```python
from build123d import *

# Parameters (mm, degrees)
F0_R     = 14
F1_DEPTH = 32
F2_DEPTH = 10
F3_D     = 16
F3_DEPTH = 50
F3_TIP   = 4.8068849522
F4_D     = 16
F4_DEPTH = 50
F4_TIP   = 4.8068849522


with BuildPart() as f1:
    # F0 (on Front) → F1 (new body)
    with BuildSketch(Plane.XZ):
        Circle(F0_R)
    extrude(amount=-F1_DEPTH)

    # F0 (on Front) → F2 (join)
    with BuildSketch(Plane.XZ):
        with BuildLine():
            Line((20, -13.2664991614), (20, 13.2664991614))
            ThreePointArc((20, 13.2664991614), (0, 24), (-20, 13.2664991614))
            Line((-20, 13.2664991614), (-20, -13.2664991614))
            ThreePointArc((-20, -13.2664991614), (0, -24), (20, -13.2664991614))
        make_face()
        with BuildLine():
            ThreePointArc((15.2337502822, 11.3548602959), (18.0338744501, 5.981586104), (19, 0))
            ThreePointArc((19, 0), (18.0338744501, -5.981586104), (15.2337502822, -11.3548602959))
            ThreePointArc((15.2337502822, -11.3548602959), (15.9359270771, -12.2913470597), (16.1850288425, -13.4350288425))
            ThreePointArc((16.1850288425, -13.4350288425), (14.3947257991, -16.0121360874), (11.3548602959, -15.2337502822))
            ThreePointArc((11.3548602959, -15.2337502822), (7.2709852149, -17.5537111177), (2.7427894128, -18.8009868421))
            ThreePointArc((2.7427894128, -18.8009868421), (2.748196762, -18.9004281295), (2.75, -19))
            ThreePointArc((2.75, -19), (-0.0995718705, -21.748196762), (-2.7427894128, -18.8009868421))
            ThreePointArc((-2.7427894128, -18.8009868421), (-7.2709852149, -17.5537111177), (-11.3548602959, -15.2337502822))
            ThreePointArc((-11.3548602959, -15.2337502822), (-15.3795724908, -15.3795724908), (-15.2337502822, -11.3548602959))
            ThreePointArc((-15.2337502822, -11.3548602959), (-19, 0), (-15.2337502822, 11.3548602959))
            ThreePointArc((-15.2337502822, 11.3548602959), (-15.3795724908, 15.3795724908), (-11.3548602959, 15.2337502822))
            ThreePointArc((-11.3548602959, 15.2337502822), (-7.2709852149, 17.5537111177), (-2.7427894128, 18.8009868421))
            ThreePointArc((-2.7427894128, 18.8009868421), (-0.0995718705, 21.748196762), (2.75, 19))
            ThreePointArc((2.75, 19), (2.748196762, 18.9004281295), (2.7427894128, 18.8009868421))
            ThreePointArc((2.7427894128, 18.8009868421), (7.2709852149, 17.5537111177), (11.3548602959, 15.2337502822))
            ThreePointArc((11.3548602959, 15.2337502822), (14.3947257991, 16.0121360874), (16.1850288425, 13.4350288425))
            ThreePointArc((16.1850288425, 13.4350288425), (15.9359270771, 12.2913470597), (15.2337502822, 11.3548602959))
        make_face(mode=Mode.SUBTRACT)
        with BuildLine():
            ThreePointArc((15.2337502822, -11.3548602959), (18.0338744501, -5.981586104), (19, 0))
            ThreePointArc((19, 0), (18.0338744501, 5.981586104), (15.2337502822, 11.3548602959))
            ThreePointArc((15.2337502822, 11.3548602959), (11.4904851943, 11.4904851943), (11.3548602959, 15.2337502822))
            ThreePointArc((11.3548602959, 15.2337502822), (7.2709852149, 17.5537111177), (2.7427894128, 18.8009868421))
            ThreePointArc((2.7427894128, 18.8009868421), (0, 16.25), (-2.7427894128, 18.8009868421))
            ThreePointArc((-2.7427894128, 18.8009868421), (-7.2709852149, 17.5537111177), (-11.3548602959, 15.2337502822))
            ThreePointArc((-11.3548602959, 15.2337502822), (-10.8579215977, 14.3947257991), (-10.6850288425, 13.4350288425))
            ThreePointArc((-10.6850288425, 13.4350288425), (-12.2913470597, 10.934130608), (-15.2337502822, 11.3548602959))
            ThreePointArc((-15.2337502822, 11.3548602959), (-19, 0), (-15.2337502822, -11.3548602959))
            ThreePointArc((-15.2337502822, -11.3548602959), (-12.2913470597, -10.934130608), (-10.6850288425, -13.4350288425))
            ThreePointArc((-10.6850288425, -13.4350288425), (-10.8579215977, -14.3947257991), (-11.3548602959, -15.2337502822))
            ThreePointArc((-11.3548602959, -15.2337502822), (-7.2709852149, -17.5537111177), (-2.7427894128, -18.8009868421))
            ThreePointArc((-2.7427894128, -18.8009868421), (0, -16.25), (2.7427894128, -18.8009868421))
            ThreePointArc((2.7427894128, -18.8009868421), (7.2709852149, -17.5537111177), (11.3548602959, -15.2337502822))
            ThreePointArc((11.3548602959, -15.2337502822), (11.4904851943, -11.4904851943), (15.2337502822, -11.3548602959))
        make_face()
        Circle(F0_R, mode=Mode.SUBTRACT)
        Circle(F0_R)
    extrude(amount=F2_DEPTH)

    # F3 (one way)
    with BuildSketch(Plane(origin=(0, 0, 0), x_dir=(1, 0, 0), z_dir=(0, 1, 0))):
        with Locations((0, 0)):
            Circle(F3_D / 2)
    extrude(amount=-F3_DEPTH, mode=Mode.SUBTRACT)
    with Locations(Plane(origin=(0, 0, 0), x_dir=(1, 0, 0), z_dir=(0, 1, 0))):
        with Locations((0, 0)):
            with Locations((0, 0, -(F3_DEPTH + F3_TIP / 2))):  # 118° drill point
                Cone(0, F3_D / 2, F3_TIP, mode=Mode.SUBTRACT)

    # F4
    with Locations(Plane.XZ):
        with Locations((0, 0)):
            Hole(F4_D / 2, depth=F4_DEPTH)
            with Locations((0, 0, -(F4_DEPTH + F4_TIP / 2))):  # 118° drill point
                Cone(0, F4_D / 2, F4_TIP, mode=Mode.SUBTRACT)


solid = f1.part
```
Input: part model. Units: mm. Frame: model coordinates. A direction names the side the tool comes from. Round coordinates to 2 decimals unless told otherwise and drop trailing zeros. Loops run counter-clockwise (first coordinate to the right, second up) from the corner with the lowest first, then second, coordinate; pieces in that order, holes last. Notation, with made-up numbers: (69, 51) -> (123, 51) arc R12 cw to (123, 74) -> close; hole circle Ø6 at (34.5, 80). An arc over 180 degrees is marked (long way). One line per item, written item: value.
(1) Section D-D (z = 12). Return the cut outline in (x, y), plus the area to 3 significant figures.
Geometry check:
outline: (-20, -10) -> (-15.78, -10) -> (-15.78, 0) -> (-20, 0) -> close; (-11.09, -10) -> (11.09, -10) -> (11.09, 0) -> (7.21, 0) -> (7.21, 32) -> (-7.21, 32) -> (-7.21, 0) -> (-11.09, 0) -> close; (15.78, -10) -> (20, -10) -> (20, 0) -> (15.78, 0) -> close
area: 768 mm2
(2) Section B-B (z = -1). Return the cut outline in (x, y).
Geometry check:
outline: (-20, -10) -> (-7.94, -10) -> (-7.94, 32) -> (-13.96, 32) -> (-13.96, 0) -> (-20, 0) -> close; (7.94, -10) -> (20, -10) -> (20, 0) -> (13.96, 0) -> (13.96, 32) -> (7.94, 32) -> close
(3) Pin query (flat end, axial travel): pin 1 (5 mm diameter, centred on x = 6.5, y = 11.5, fed in from -Z); pin 2 (4.5 mm diameter, centred on x = 13.44, z = 13.44, fed in from -Y); pin 3 (2 mm diameter, centred on x = -2.5, z = 17, fed in from +Y); pin 4 (1.5 mm diameter, centred on y = 21.5, z = 7.5, fed in from +X). Return the tip coordinate at first contact, or that it passes through.
Geometry check:
pin 1: z = -13.42
pin 2: through
pin 3: y = 0
pin 4: x = 12.27
(4) Section C-C (y = -5.5). Return the cut outline in (x, z), plus the area to 3 significant figures.
Geometry check:
outline: (-20, -13.27) arc R24 ccw to (20, -13.27) -> (20, 13.27) arc R24 ccw to (-20, 13.27) -> close; hole circle Ø5.5 at (-13.44, -13.44); hole circle Ø5.5 at (-13.44, 13.44); hole circle Ø16 at (0, 0); hole circle Ø5.5 at (0, -19); hole circle Ø5.5 at (0, 19); hole circle Ø5.5 at (13.44, -13.44); hole circle Ø5.5 at (13.44, 13.44)
area: 1,320 mm2
(5) Material intervals for line 1 (X direction, y = -2, z = -13); line 2 (Z direction, x = -11.5, y = -4.5); line 3 (Z direction, x = 0, y = 11.5), sorted ascending. Write a range as [from, to].
Geometry check:
line 1: [-20, -16.15], [-10.72, 10.72], [16.15, 20]
line 2: [-21.07, -15.39], [-11.48, 11.48], [15.39, 21.07]
line 3: [-14, -8], [8, 14]
(6) Set-up query: faces 1 (the face through (9, -10, 0)), 2 (the face through (-9, 0, 11)). Return all of +Z, -Z, +X, -X, +Y, -Y with unobstructed straight access to the full face (end or side cutting, diameter ignored); none if empty.
Geometry check:
face 1: +Z, -Z, +X, -X, -Y
face 2: +Y
(7) Mould query, pull axis Z, two halves, no side actions, for faces 3 (the face through (0, -5, 24)), 4 (the face through (12.932, 15.776, -5.362)), 5 (the face through (0, -5, -24)), 6 (the face through (20, -5, 0)). Classes: pulls with the +Z half, pulls with the -Z half, needs draft (parallel to the pull), parting line crosses it, or undercut.
Geometry check:
face 3: pulls with the +Z half
face 4: parting line crosses it
face 5: pulls with the -Z half
face 6: needs draft
(8) Section A-A (x = 0). Return the cut outline in (y, z), plus the area to 3 significant figures.
Geometry check:
outline: (-10, -24) -> (0, -24) -> (0, -21.75) -> (-10, -21.75) -> close; (-10, -16.25) -> (0, -16.25) -> (0, -14) -> (32, -14) -> (32, -8) -> (-10, -8) -> close; (-10, 8) -> (32, 8) -> (32, 14) -> (0, 14) -> (0, 16.25) -> (-10, 16.25) -> close; (-10, 21.75) -> (0, 21.75) -> (0, 24) -> (-10, 24) -> close
area: 594 mm2
